```python
from build123d import *

# Parameters (mm, degrees)
F1_DEPTH = 15.24
F3_DEPTH = 15.24
F5_D     = 7
F6_R     = 5.08
F7_R     = 2.54
F8_R     = 0.762
F9_R     = 0.254


with BuildPart() as f1:
    # F0 (on Front) → F1 (new body)
    with BuildSketch(Plane.XZ):
        with BuildLine():
            ThreePointArc((-5.4838847455, 13.5661152545), (-9.2757152012, 3.8154394137), (-13.9029439924, 13.1985311894))
            Line((-13.9029439924, 13.1985311894), (-15.8486968779, 14.831211718))
            ThreePointArc((-15.8486968779, 14.831211718), (-9.1649219573, 1.2778569308), (-3.6878335213, 15.3621664787))
            Line((-3.6878335213, 15.3621664787), (-5.4838847455, 13.5661152545))
        make_face()
    extrude(amount=F1_DEPTH)



with BuildPart() as f1b:
    # F0 (on Front) → F1, piece 2 (new body)
    with BuildSketch(Plane.XZ):
        with BuildLine():
            ThreePointArc((13.9452403049, 12.9163381462), (9.2059751792, 3.5893330735), (5.531186829, 13.3847191373))
            Line((5.531186829, 13.3847191373), (3.7567731907, 15.2021503575))
            ThreePointArc((3.7567731907, 15.2021503575), (9.0648008077, 1.0532593765), (15.9104059892, 14.525600037))
            Line((15.9104059892, 14.525600037), (13.9452403049, 12.9163381462))
        make_face()
    extrude(amount=F1_DEPTH)


with BuildPart() as f1_1:
    add(f1.part)

    add(f1b.part)  # F3 merges F1b
    # F2 (on Front) → F3 (join)
    with BuildSketch(Plane.XZ):
        Polygon((12.2539751792, 1.7834394137), (-19.304, 1.7834394137), (-19.304, 16.609211718), (-39.624, 16.609211718), (-39.624, 11.021211718), (-24.384, 11.021211718), (-24.384, -2.0265605863), (7.7133939915, -2.0265605863), align=None)
    extrude(amount=F3_DEPTH)

    # F5 (through all)
    with Locations(Plane(origin=(0, 0, 11.021211718), x_dir=(1, 0, 0), z_dir=(0, 0, -1))):
        with Locations((-32.004, 7.62)):
            Hole(F5_D / 2)

    # F6
    f6_edges = [f1_1.edges().sort_by_distance(p)[0] for p in [
        (-39.624, -15.24, 13.815212),
        (-39.624, 0, 13.815212),
        (-24.384, -7.62, -2.026561),
        (11.72475, -7.62, 1.339367),
        (7.713394, -7.62, -2.026561),
    ]]
    fillet(f6_edges, radius=F6_R)

    # F7
    f7_edges = [f1_1.edges().sort_by_distance(p)[0] for p in [
        (-19.304, -7.62, 16.609212),
        (-19.304, -7.62, 1.783439),
        (-13.902944, -7.62, 13.198531),
        (-5.483885, -7.62, 13.566115),
        (5.531187, -7.62, 13.384719),
        (13.94524, -7.62, 12.916338),
    ]]
    fillet(f7_edges, radius=F7_R)

    # F8
    f8_edges = [f1_1.edges().sort_by_distance(p)[0] for p in [
        (-15.848697, -7.62, 14.831212),
        (-3.687834, -7.62, 15.362166),
        (3.756773, -7.62, 15.20215),
        (15.910406, -7.62, 14.5256),
        (-24.384, -7.62, 11.021212),
    ]]
    fillet(f8_edges, radius=F8_R)

    # F9
    f9_edges = [f1_1.edges().sort_by_distance(p)[0] for p in [
        (-6.659121, -7.62, 1.783439),
        (-12.390879, -7.62, 1.783439),
        (6.101047, -7.62, 1.783439),
    ]]
    fillet(f9_edges, radius=F9_R)


solid = f1_1.part
```
Here's how the part is built. I have some questions about the finished solid (model axes, mm). A direction names the side the tool comes from. Give positions to 0.01 mm unless a question says otherwise; leave off trailing zeros. Write each loop counter-clockwise with the first axis right and the second up, starting at its lowest first coordinate (ties: lowest second). Pieces come first, ordered by that corner, then holes. Notation, with made-up numbers: M -20,35 L -7,35 A18 cw -7,44 Z; hole C 12,34.5 d5. An arc over 180 degrees is marked long. Put each result on its own line as item: value. Start each with the question number.
Item 1: If we section it at B-B, the plane x = -27: Write out the boundary of the cut face in (y, z), then the cut area to 3 significant figures.
Item 2: On a 3-axis mill with a long thin cutter (end or side, diameter ignored), from which of +Z, -Z, +X, -X, +Y, -Y can I reach the whole of each face in a straight line? I mean faces 1 (the flat face through (-28.6, -5.8, 16.609)), 2 (the flat face through (-36, -8, 11.021)), 3 (the flat face through (-7, -8, -2.027)), 4 (the cylindrical face through (-20.068, -7.727, 15.885)), 5 (the flat face through (-15, -8, 1.783)). Say none if no direction works.
Item 3: Thinking about a two-plate mould opening in Z: for faces 6 (the cylindrical face through (-17.56, -7.51, 7.63)), 7 (the cylindrical face through (7.58, -7.73, -1.73)), 8 (the cylindrical face through (4.757, -7.727, 13.234)), 9 (the cylindrical face through (-38.18, -13.71, 13.78)), which applies, +Z half, -Z half, draft (parallel to the pull), parting line (faces both ways), or undercut?
Item 4: Will these pins go through, and if not, where does the flat tip stop? pin 1 (1.6 mm diameter, centred on x = -15.5, y = -10.5, fed in from +Z); pin 2 (1.5 mm diameter, centred on x = -1.5, z = 6, fed in from -Y); pin 3 (6 mm diameter, centred on x = 0.5, y = -4.5, fed in from +Z); pin 4 (1 mm diameter, centred on x = -2, y = -7.5, fed in from +Z).
Item 5: I need wall thicknesses on L1, parallel to X at y = -1.5, z = 2.5; L2, parallel to X at y = -8.5, z = 11.5; L3, parallel to X at y = -2, z = 8.5. Which ranges of each line are inside material? Lowest first, please. Write a range as from..to.
Item 6: If we section it at A-A, the plane z = 9: Write out the boundary of the cut face in (x, y), then the cut area to 3 significant figures.
Values:
1. outline: M -15.24,11.02 L 0,11.02 L 0,16.61 L -15.24,16.61 Z
1. area: 85.2 mm²
2. face 1: +Z, +X, -X, +Y, -Y
2. face 2: -Z, -X, +Y, -Y
2. face 3: -Z, +X, -X, +Y, -Y
2. face 4: +Z, +Y, -Y
2. face 5: +Y, -Y
3. face 6: undercut
3. face 7: -Z half
3. face 8: undercut
3. face 9: draft
4. pin 1: z = 14.46
4. pin 2: y = -15.24
4. pin 3: z = 14.78
4. pin 4: z = 13.86
5. L1: -24.35..-18.53, -13.86..-5.19, 4.84..14.21
5. L2: -39.62..-35.39, -28.62..-19.3, -17.54..-14.89, -4.16..-1.51, 1.57..4.25, 14.8..17.48
5. L3: -24.38..-19.3, -17.72..-15.15, -3.9..-1.33, 1.31..3.86, 15.18..17.74
6. outline: M -24.38,-15.24 L -19.3,-15.24 L -19.3,0 L -24.38,0 Z; M -17.76,-15.24 L -15.22,-15.24 L -15.22,0 L -17.76,0 Z; M -3.83,-15.24 L -1.29,-15.24 L -1.29,0 L -3.83,0 Z; M 1.27,-15.24 L 3.82,-15.24 L 3.82,0 L 1.27,0 Z; M 15.23,-15.24 L 17.77,-15.24 L 17.77,0 L 15.23,0 Z
6. area: 233 mm²
